The model under review builds one solid part; all positions refer to its coordinate system, in mm. Face numbers are marked on the shaded views. A direction names the side the tool comes from. Round coordinates to 2 decimals unless told otherwise and drop trailing zeros. Write each loop counter-clockwise with the first axis right and the second up, starting at its lowest first coordinate (ties: lowest second). Pieces come first, ordered by that corner, then holes. Notation, with made-up numbers: (-33, -32) - (-21, -32) arc R25 cw to (-21, 4) - close; hole circle Ø4 at (-35.75, 73.25). An arc over 180 degrees is marked (long way). Write each question's results on one line, items separated by ' | '.
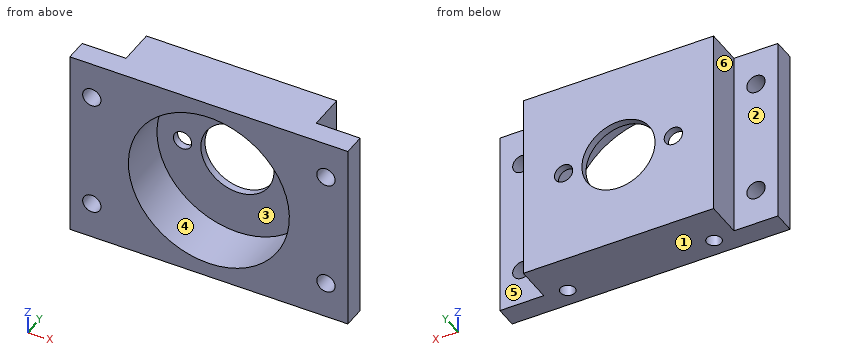
```python
from build123d import *

# Parameters (mm, degrees)
BOSS_EXTRUDE1_DEPTH = 26
SKETCH2_R           = 5
SKETCH2_R_2         = 1.25
CUT_EXTRUDE1_DEPTH  = 47.733285782
SKETCH3_R           = 11
CUT_EXTRUDE2_DEPTH  = 7
SKETCH5_R           = 1
CUT_EXTRUDE7_DEPTH  = 6


with BuildPart() as part:
    # Sketch1 → Boss-Extrude1 (new body)
    with BuildSketch(Plane.XY):
        Polygon((0, 0), (8, 0), (30, 0), (38, 0), (38, 3), (32, 3), (32, 8), (6, 8), (6, 3), (0, 3), align=None)
    extrude(amount=BOSS_EXTRUDE1_DEPTH)

    # Sketch2 → Cut-Extrude1 (cut, through all)
    with BuildSketch(Plane(origin=(0, 8, 0), x_dir=(1, 0, 0), z_dir=(0, 1, 0))):
        with Locations(Location((19, -13, 0), (0, 0, 180))):
            Circle(SKETCH2_R)
        with Locations(Location((11.5, -13, 0), (0, 0, 180))):
            Circle(SKETCH2_R_2)
        with Locations(Location((26.5, -13, 0), (0, 0, 180))):
            Circle(SKETCH2_R_2)
        with Locations(Location((3, -21, 0), (0, 0, 180))):
            Circle(SKETCH2_R_2)
        with Locations(Location((3, -5, 0), (0, 0, 180))):
            Circle(SKETCH2_R_2)
        with Locations(Location((35, -21, 0), (0, 0, 180))):
            Circle(SKETCH2_R_2)
        with Locations(Location((35, -5, 0), (0, 0, 180))):
            Circle(SKETCH2_R_2)
    extrude(amount=-CUT_EXTRUDE1_DEPTH, mode=Mode.SUBTRACT)

    # Sketch3 → Cut-Extrude2 (cut)
    with BuildSketch(Plane.XZ):
        with Locations(Location((19, 13, 0), (0, 0, 270))):
            Circle(SKETCH3_R)
    extrude(amount=-CUT_EXTRUDE2_DEPTH, mode=Mode.SUBTRACT)

    # Sketch5 → Cut-Extrude7 (cut)
    with BuildSketch(Plane(origin=(0, 0, 0), x_dir=(-1, 0, 0), z_dir=(0, 0, -1))):
        with Locations((-29, 2.5)):
            Circle(SKETCH5_R)
        with Locations((-9, 2.5)):
            Circle(SKETCH5_R)
    extrude(amount=-CUT_EXTRUDE7_DEPTH, mode=Mode.SUBTRACT)


solid = part.part
```
Q1. We need section A-A (z = 5). State the section outline as (x, y) points, plus the area to 3 significant figures.
Evaluation:
outline: (0, 0) - (1.75, 0) - (1.75, 3) - (0, 3) - close; (4.25, 0) - (11.45, 0) - (11.45, 7) - (26.55, 7) - (26.55, 0) - (33.75, 0) - (33.75, 3) - (32, 3) - (32, 8) - (6, 8) - (6, 3) - (4.25, 3) - close; (36.25, 0) - (38, 0) - (38, 3) - (36.25, 3) - close; hole circle Ø2 at (9, 2.5); hole circle Ø2 at (29, 2.5) | area: 117 mm^2
Q2. The part is to be moulded in two halves that separate along X. For the marked faces 4, 5 and 6, say which applies: released by +X, released by -X, zero draft, split by the parting line, or undercut.
Evaluation:
face 4: undercut | face 5: zero draft | face 6: released by -X
Q3. We need section D-D (y = 2.5). State the section outline as (x, z) points, plus the area to 3 significant figures.
Evaluation:
outline: (0, 0) - (8, 0) - (8, 6) - (10, 6) - (10, 0) - (28, 0) - (28, 6) - (30, 6) - (30, 0) - (38, 0) - (38, 26) - (0, 26) - close; hole circle Ø2.5 at (3, 5); hole circle Ø2.5 at (3, 21); hole circle Ø22 at (19, 13); hole circle Ø2.5 at (35, 5); hole circle Ø2.5 at (35, 21) | area: 564 mm^2
Q4. We need section C-C (z = 13). State the section outline as (x, y) points.
Evaluation:
outline: (0, 0) - (8, 0) - (8, 7) - (10.25, 7) - (10.25, 8) - (6, 8) - (6, 3) - (0, 3) - close; (12.75, 7) - (14, 7) - (14, 8) - (12.75, 8) - close; (24, 7) - (25.25, 7) - (25.25, 8) - (24, 8) - close; (27.75, 7) - (30, 7) - (30, 0) - (38, 0) - (38, 3) - (32, 3) - (32, 8) - (27.75, 8) - close
Q5. Insertion check: P1, Ø11.5, axis at x = 19, z = 13, coming from the -Y side; P2, Ø2, axis at y = 5.5, z = 13, coming from the +X side; P3, Ø2, axis at x = 26.5, z = 13, coming from the +Y side; P4, Ø3, axis at x = 3, z = 21, coming from the +Y side. Each pin has a flat end and moves straight along its axis. Give the tip position at first contact, or say it passes through.
Evaluation:
P1: stops at y = 7 | P2: stops at x = 32 | P3: passes through | P4: stops at y = 3
Q6. Tool access review of the marked faces 1, 2 and 3: name each direction out of +Z, -Z, +X, -X, +Y, -Y from which nothing blocks a thin tool from reaching the whole face with its end or side.
Evaluation:
face 1: -Z, +X, -X, +Y, -Y | face 2: +Z, -Z, -X, +Y | face 3: -Y
Q7. We need section B-B (x = 3). State the section outline as (y, z) points, plus the area to 3 significant figures.
Evaluation:
outline: (0, 0) - (3, 0) - (3, 3.75) - (0, 3.75) - close; (0, 6.25) - (3, 6.25) - (3, 19.75) - (0, 19.75) - close; (0, 22.25) - (3, 22.25) - (3, 26) - (0, 26) - close | area: 63.0 mm^2
Q8. For probe 1 along Z at (x, y) = (26.5, 7.2); probe 2 along Z at (x, y) = (19, 7.2); probe 3 along X at (y, z) = (0.5, 4.75), list the stretches that pass through material, from the lowest coordinate up.
Evaluation:
probe 1: z = 0 to 11.75, 14.25 to 26 | probe 2: z = 0 to 8, 18 to 26 | probe 3: x = 0 to 1.78, 4.22 to 11.72, 26.28 to 33.78, 36.22 to 38
